Part model, mm, in its own coordinate system. A direction names the side the tool comes from. Give positions to 0.01 mm unless a question says otherwise; leave off trailing zeros. Write each loop counter-clockwise with the first axis right and the second up, starting at its lowest first coordinate (ties: lowest second). Pieces come first, ordered by that corner, then holes. Notation, with made-up numbers: M 65,-9 L 108,-9 A15 cw 108,-2 Z; hole C 38,36.5 d5. An arc over 180 degrees is marked long. Use a Markdown table: item, result.
```python
from build123d import *

# Parameters (mm, degrees)
SKETCH1_W           = 660
SKETCH1_H           = 420
BOSS_EXTRUDE1_DEPTH = 120
SKETCH2_W           = 120
SKETCH2_H           = 420
BOSS_EXTRUDE2_DEPTH = 480
FILLET1_RADIUS      = 210
FILLET1_LENGTH      = 120
CHAMFER1_START      = 376.454614173
CHAMFER1_OUTLINE_W  = 172
CHAMFER1_OUTLINE_H  = 120
CHAMFER1_DEPTH      = 85.545385827
CHAMFER2_START      = 616.17299772
CHAMFER2_OUTLINE_W  = 173
CHAMFER2_OUTLINE_H  = 120
CHAMFER2_DEPTH      = 85.82700228
SKETCH4_W           = 120
SKETCH4_H           = 420
BOSS_EXTRUDE3_DEPTH = 540
CUT_EXTRUDE1_DEPTH  = 480


with BuildPart() as part:
    # Sketch1 → Boss-Extrude1 (new body)
    with BuildSketch(Plane(origin=(0, 0, 0), x_dir=(1, 0, 0), z_dir=(0, 1, 0))):
        with Locations((281.893715562, 169.506494581)):
            Rectangle(SKETCH1_W, SKETCH1_H)
    extrude(amount=BOSS_EXTRUDE1_DEPTH)

    # Sketch2 → Boss-Extrude2 (add)
    with BuildSketch(Plane(origin=(0, 120, 0), x_dir=(1, 0, 0), z_dir=(0, 1, 0))):
        with Locations((11.893715562, 169.506494581)):
            Rectangle(SKETCH2_W, SKETCH2_H)
    extrude(amount=BOSS_EXTRUDE2_DEPTH)

    # Fillet1: full round fillet: the end face becomes a half cylinder, R = half its width
    fillet1_face = Plane((11.893715562, 600, -169.506494581), x_dir=(1, 0, 0), z_dir=(0, 1, 0))  # on the end face: x along it, z out of the body
    fillet1_slab = fillet1_face.offset(-FILLET1_RADIUS / 2) * Box(FILLET1_LENGTH, 2 * FILLET1_RADIUS, FILLET1_RADIUS, mode=Mode.PRIVATE)  # the body's end, R deep
    fillet1_round = Plane((11.893715562, 390, -169.506494581), x_dir=(0, 1, 0), z_dir=(1, 0, 0)) * Cylinder(FILLET1_RADIUS, FILLET1_LENGTH, mode=Mode.PRIVATE)  # its axis R under the face
    add(fillet1_slab - fillet1_round, mode=Mode.SUBTRACT)

    # Chamfer1: read off the stored shape, not the designer's step
    # Chamfer1 outline → Chamfer1 (cut)
    with BuildSketch(Plane(origin=(0, 0, 0), x_dir=(0.7071067811865471, 0, -0.707106781186548), z_dir=(0.707106781186548, 0, 0.707106781186547)).offset(CHAMFER1_START)):
        with Locations((404, 60)):
            Rectangle(CHAMFER1_OUTLINE_W, CHAMFER1_OUTLINE_H)
    extrude(amount=CHAMFER1_DEPTH, mode=Mode.SUBTRACT)

    # Chamfer2: read off the stored shape, not the designer's step
    # Chamfer2 outline → Chamfer2 (cut)
    with BuildSketch(Plane(origin=(0, 0, 0), x_dir=(0.707106781186548, 0, 0.707106781186547), z_dir=(0.707106781186547, 0, -0.707106781186548)).offset(CHAMFER2_START)):
        with Locations((164.5, -60)):
            Rectangle(CHAMFER2_OUTLINE_W, CHAMFER2_OUTLINE_H)
    extrude(amount=CHAMFER2_DEPTH, mode=Mode.SUBTRACT)

    # Sketch4 → Boss-Extrude3 (add)
    with BuildSketch(Plane(origin=(71.893715562, 0, 0), x_dir=(0, 0, -1), z_dir=(1, 0, 0))):
        with Locations((169.506494581, 330)):
            Rectangle(SKETCH4_W, SKETCH4_H)
    extrude(amount=BOSS_EXTRUDE3_DEPTH)

    # Sketch7 → Cut-Extrude1 (cut)
    with BuildSketch(Plane.XY.offset(-109.506494581)):
        Polygon((71.893715562, 540), (611.893715562, 120), (611.893715562, 540), align=None)
    extrude(amount=-CUT_EXTRUDE1_DEPTH, mode=Mode.SUBTRACT)


solid = part.part
```
1. Drop flat-ended pins along their axis: P1, Ø12, axis at x = 260.5, z = -216.5, coming from the +Y side; P2, Ø8, axis at y = 534.5, z = -151.5, coming from the +X side; P3, Ø6, axis at y = 201, z = -144, coming from the +X side. Give the stop position or say it passes through.
Findings below:
| item | result |
|---|---|
| P1 | y = 397.97 |
| P2 | x = 84.11 |
| P3 | x = 511.61 |
2. Tool access for faces 1 (the flat face through (71.894, 357, -260)), 2 (the flat face through (338, 120, -36)), 3 (the flat face through (158, 106, 40.494)), 4 (the flat face through (551.1, 59.2, -320.3)), 5 (the flat face through (278, 280, -229.506)): list every direction of +Z, -Z, +X, -X, +Y, -Y with a clear straight run to the whole face (end or side of a thin tool).
Findings below:
| item | result |
|---|---|
| face 1 | +X, +Y |
| face 2 | +Z, +X, +Y |
| face 3 | +Z, +X, -X, +Y, -Y |
| face 4 | -Z, +X, +Y, -Y |
| face 5 | -Z, +X, +Y |
3. Drill centre lines: L1, parallel to X at y = 404, z = -295; L2, parallel to Z at x = 134.5, y = 306; L3, parallel to Y at x = 402.5, z = -283.5. Where is each one in solid material? Low to high.
Findings below:
| item | result |
|---|---|
| L1 | -48.11 to 71.89 |
| L2 | -229.51 to -109.51 |
| L3 | 0 to 120 |
4. Cut at D-D, the plane z = -283. Give the cut face in (x, y), then the cut area to 3 significant figures.
Findings below:
| item | result |
|---|---|
| outline | M -48.11,0 L 588.4,0 L 588.4,120 L 71.89,120 L 71.89,566.69 L -48.11,566.69 Z |
| area | 130,000 mm2 |
5. Cut at C-C, the plane y = 355.5. Give the cut face in (x, z).
Findings below:
| item | result |
|---|---|
| outline | M -48.11,-379.51 L 71.89,-379.51 L 71.89,-229.51 L 309.11,-229.51 L 309.11,-109.51 L 71.89,-109.51 L 71.89,40.49 L -48.11,40.49 Z |
6. Cut at B-B, the plane z = -210.5. Give the cut face in (x, y), then the cut area to 3 significant figures.
Findings below:
| item | result |
|---|---|
| outline | M -48.11,0 L 611.89,0 L 611.89,120 L 71.89,540 L 71.89,595.96 L -48.11,595.96 Z |
| area | 250,000 mm2 |
7. Cut at A-A, the plane x = 373.5. Give the cut face in (y, z), then the cut area to 4 significant figures.
Findings below:
| item | result |
|---|---|
| outline | M 0,-379.51 L 120,-379.51 L 120,-229.51 L 305.42,-229.51 L 305.42,-109.51 L 120,-109.51 L 120,40.49 L 0,40.49 Z |
| area | 72,650 mm2 |
